Check sheet for the modelled part. Datum: model origin and axes. Units: mm. Round coordinates to 2 decimals unless told otherwise and drop trailing zeros. Write each loop counter-clockwise with the first axis right and the second up, starting at its lowest first coordinate (ties: lowest second). Pieces come first, ordered by that corner, then holes. Notation, with made-up numbers: M 87.25,14.5 L 118.25,14.5 A23 cw 118.25,35.5 Z; hole C -23,32 d2. An arc over 180 degrees is marked long. One line per item, written item: value.
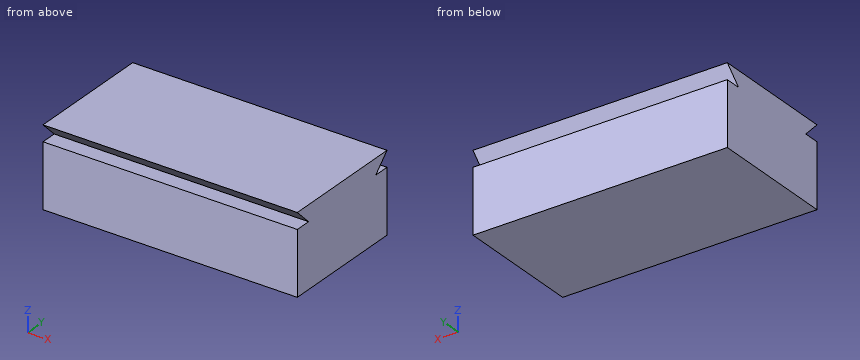
from build123d import *

# Parameters (mm, degrees)
F0_W     = 203.2
F0_H     = 101.6
F1_DEPTH = 63.5
F3_DEPTH = 215.9
F5_DEPTH = 215.9


with BuildPart() as f1:
    # F0 (on Top) → F1 (new body)
    with BuildSketch(Plane.XY):
        Rectangle(F0_W, F0_H)
    extrude(amount=F1_DEPTH)

    # F2 (on face) → F3 (cut)
    with BuildSketch(Plane.YZ.offset(101.6)):
        Polygon((50.8, 50.8), (50.8, 63.5), (38.1, 50.8), align=None)
    extrude(amount=-F3_DEPTH, mode=Mode.SUBTRACT)

    # F4 (on face) → F5 (cut)
    with BuildSketch(Plane.YZ.offset(101.6)):
        Polygon((-38.1, 50.8), (-50.8, 63.5), (-50.8, 50.8), align=None)
    extrude(amount=-F5_DEPTH, mode=Mode.SUBTRACT)


solid = f1.part
Q1. Scan lines: line 1 (Z direction, x = 86, y = 46); line 2 (Z direction, x = -65, y = 44). Record each from-to range of solid material in increasing order. Write a range as [from, to].
Completed:
line 1: [0, 50.8], [58.7, 63.5]
line 2: [0, 50.8], [56.7, 63.5]
Q2. Depth check by flat-ended pin: P1, Ø3, axis at x = -28, y = -4, coming from the -Z side. Enter the tip coordinate at first touch or a pass-through.
Completed:
P1: z = 0
Q3. Sectioned sample at A-A on y = -45. Enter the section's corners in (x, z), and give its area (3 significant figures).
Completed:
outline: M -101.6,0 L 101.6,0 L 101.6,50.8 L -101.6,50.8 Z; M -101.6,57.7 L 101.6,57.7 L 101.6,63.5 L -101.6,63.5 Z
area: 11,500 mm^2
Q4. Sectioned sample at B-B on x = 84.5. Enter the section's corners in (y, z), and give its area (3 significant figures).
Completed:
outline: M -50.8,0 L 50.8,0 L 50.8,50.8 L 38.1,50.8 L 50.8,63.5 L -50.8,63.5 L -38.1,50.8 L -50.8,50.8 Z
area: 6,290 mm^2
